from build123d import *

# Parameters (mm, degrees)
SKETCH1_W           = 40
SKETCH1_H           = 40
SKETCH1_R           = 1.8
SKETCH1_R_2         = 18.484463189
BOSS_EXTRUDE1_DEPTH = 20
FILLET1_R           = 3


with BuildPart() as part:
    # Sketch1 → Boss-Extrude1 (new body)
    with BuildSketch(Plane.XY):
        Rectangle(SKETCH1_W, SKETCH1_H)
        with Locations((-16, 16)):
            Circle(SKETCH1_R, mode=Mode.SUBTRACT)
        with Locations((16, 16)):
            Circle(SKETCH1_R, mode=Mode.SUBTRACT)
        with Locations((16, -16)):
            Circle(SKETCH1_R, mode=Mode.SUBTRACT)
        with Locations((-16, -16)):
            Circle(SKETCH1_R, mode=Mode.SUBTRACT)
        Circle(SKETCH1_R_2, mode=Mode.SUBTRACT)
    extrude(amount=BOSS_EXTRUDE1_DEPTH)

    # Fillet1
    fillet1_edges = [part.edges().sort_by_distance(p)[0] for p in [
        (20, -20, 10),
        (-20, -20, 10),
        (-20, 20, 10),
        (20, 20, 10),
    ]]
    fillet(fillet1_edges, radius=FILLET1_R)


solid = part.part
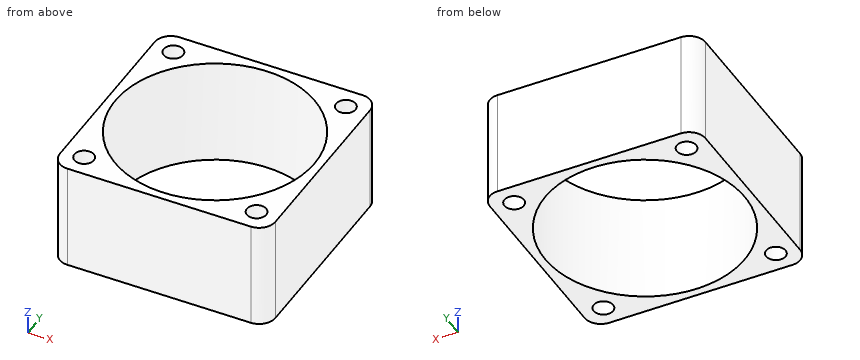
Read the model definition and answer for the solid it produces. Units are mm, in the model's axes. Round coordinates to 2 decimals unless told otherwise and drop trailing zeros. Order: outer loops, then holes, each group sorted by start corner. A loop starts at its lowest first (then second) coordinate and runs counter-clockwise, first axis right, second up. Notation, with made-up numbers: (56, 45) - (69, 45) arc R21 ccw to (69, 54) - close; hole circle Ø4 at (-25, -4). An arc over 180 degrees is marked (long way). Use one line per item in the form item = value. Start each with the question number.
(1) The part is cut by section D-D (y = 16). Give the vertices of the cut face in (x, z).
(2) The part is cut by section C-C (z = 4). Give the vertices of the cut face in (x, y), then the cut area to 3 significant figures.
(3) The part is cut by section A-A (x = 0). Give the vertices of the cut face in (y, z).
(4) Flat-ended cylindrical pins translate along their axes: pin 1 Ø5 at (x, y) = (-15, 4) entering from +Z; pin 2 Ø12 at (x, y) = (-14, 2) entering from -Z. Find the tip coordinate at first contact, or state that the pin passes through.
(5) The part is cut by section B-B (y = -12.5). Give the vertices of the cut face in (x, z).
(6) Find the intervals of material crossed by line 1 along Y through (x, z) = (16, 5.75); line 2 along X through (y, z) = (16.5, 13); line 3 along X through (y, z) = (17, 1.5), in increasing order. Write a range as from..to.
Checked values:
q1.outline = (-20, 0) - (-17.8, 0) - (-17.8, 20) - (-20, 20) - close; (-14.2, 0) - (-9.26, 0) - (-9.26, 20) - (-14.2, 20) - close; (9.26, 0) - (14.2, 0) - (14.2, 20) - (9.26, 20) - close; (17.8, 0) - (20, 0) - (20, 20) - (17.8, 20) - close
q2.outline = (-20, -17) arc R3 ccw to (-17, -20) - (17, -20) arc R3 ccw to (20, -17) - (20, 17) arc R3 ccw to (17, 20) - (-17, 20) arc R3 ccw to (-20, 17) - close; hole circle Ø36.97 at (0, 0); hole circle Ø3.6 at (-16, -16); hole circle Ø3.6 at (-16, 16); hole circle Ø3.6 at (16, -16); hole circle Ø3.6 at (16, 16)
q2.area = 478 mm^2
q3.outline = (-20, 0) - (-18.48, 0) - (-18.48, 20) - (-20, 20) - close; (18.48, 0) - (20, 0) - (20, 20) - (18.48, 20) - close
q4.pin_1 = through
q4.pin_2 = 0
q5.outline = (-20, 0) - (-13.62, 0) - (-13.62, 20) - (-20, 20) - close; (13.62, 0) - (20, 0) - (20, 20) - (13.62, 20) - close
q6.line_1 = -20..-17.8, -14.2..-9.26, 9.26..14.2, 17.8..20
q6.line_2 = -20..-17.73, -14.27..-8.33, 8.33..14.27, 17.73..20
q6.line_3 = -20..-17.5, -14.5..-7.26, 7.26..14.5, 17.5..20
